from build123d import *

# Parameters (mm, degrees)
F0_W          = 76.2
F0_H          = 12.7
F1_DEPTH      = 19.05
F2_R          = 19.05
F3_DEPTH      = 19.05
F3_DEPTH_BACK = 8.2509537059
F4_START      = 20.9509537059
F4_DEPTH      = 23.4990462941
F5_R          = 7.9375
F6_DEPTH      = 101.6
F8_START      = 23.32678
F7_R          = 12.7
F8_DEPTH      = 6.84063


with BuildPart() as f1:
    # F0 (on Front) → F1 (new body, symmetric)
    with BuildSketch(Plane.XZ):
        with Locations((1.1919587851, 14.6009537059)):
            Rectangle(F0_W, F0_H)
    extrude(amount=F1_DEPTH, both=True)

    # F2 (on Top) → F3 (join, two sides)
    with BuildSketch(Plane.XY) as f3_sk:
        Circle(F2_R)
    extrude(amount=-F3_DEPTH)
    extrude(f3_sk.sketch, amount=F3_DEPTH_BACK)

    # F2 (on Top) → F4 (join)
    with BuildSketch(Plane.XY.offset(F4_START)):
        Circle(F2_R)
    extrude(amount=F4_DEPTH)

    # F5 (on Top) → F6 (cut, symmetric)
    with BuildSketch(Plane.XY):
        Circle(F5_R)
    extrude(amount=F6_DEPTH, both=True, mode=Mode.SUBTRACT)

    # F7 (on Top) → F8 (cut)
    with BuildSketch(Plane.XY.offset(F8_START)):
        Circle(F7_R)
    extrude(amount=F8_DEPTH, mode=Mode.SUBTRACT)


solid = f1.part
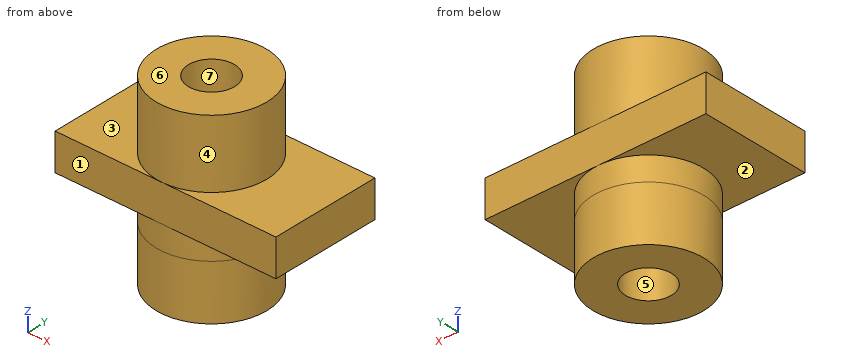
Can you work these out from the model? Positions are in its coordinate system, mm. Face numbers are marked on the shaded views. A direction names the side the tool comes from. Give positions to 0.01 mm unless a question says otherwise; leave off trailing zeros. Order: outer loops, then holes, each group sorted by start corner. A loop starts at its lowest first (then second) coordinate and runs counter-clockwise, first axis right, second up. Notation, with made-up numbers: M -33.75,8 L -7.75,8 A27 ccw -7.75,37 Z; hole C 55,67 d9. An arc over 180 degrees is marked long. Use one line per item in the form item = value. Start each with the question number.
Item 1: Will these pins go through, and if not, where does the flat tip stop? pin 1 Ø1 at (y, z) = (6.5, -1.5) entering from +X; pin 2 Ø20.5 at (x, y) = (0, 0) entering from -Z; pin 3 Ø1.5 at (y, z) = (4, 2) entering from -X; pin 4 Ø4 at (x, z) = (-16, 35) entering from +Y.
Item 2: If we section it at C-C (z = 25): Write out the boundary of the cut face in (x, y).
Item 3: If we section it at A-A (y = 3.5): Write out the boundary of the cut face in (x, z), then the cut area to 3 significant figures.
Item 4: If we section it at B-B (x = 2): Write out the boundary of the cut face in (y, z).
Item 5: We'd pull the mould along X, two halves only. Please class the marked faces 4, 5, 6 and 7: +X half, -X half, draft (parallel to the pull), parting line (faces both ways), or undercut.
Item 6: If I drill on line 1 along Y through (x, z) = (0, 11.5); line 2 along Y through (x, z) = (0, 28.5); line 3 along Z through (x, y) = (-23, -4), over which ranges is the centre line in solid material (lowest first)?
Item 7: If we section it at D-D (x = -30): Write out the boundary of the cut face in (y, z).
Item 8: For the marked faces 1, 2 and 3, which set-ups out of +Z, -Z, +X, -X, +Y, -Y let a thin tool reach every point of the face, with its end or its side?
Outcome:
q1.pin_1 = 18.08
q1.pin_2 = -19.05
q1.pin_3 = -18.77
q1.pin_4 = 12.92
q2.outline = C 0,0 d38.1; hole C 0,0 d25.4
q3.outline = M -36.91,8.25 L -18.73,8.25 L -18.73,-19.05 L -7.12,-19.05 L -7.12,23.33 L -12.21,23.33 L -12.21,30.17 L -7.12,30.17 L -7.12,44.45 L -18.73,44.45 L -18.73,20.95 L -36.91,20.95 Z; M 7.12,-19.05 L 18.73,-19.05 L 18.73,8.25 L 39.29,8.25 L 39.29,20.95 L 18.73,20.95 L 18.73,44.45 L 7.12,44.45 L 7.12,30.17 L 12.21,30.17 L 12.21,23.33 L 7.12,23.33 Z
q3.area = 1,900 mm2
q4.outline = M -19.05,8.25 L -18.94,8.25 L -18.94,-19.05 L -7.68,-19.05 L -7.68,23.33 L -12.54,23.33 L -12.54,30.17 L -7.68,30.17 L -7.68,44.45 L -18.94,44.45 L -18.94,20.95 L -19.05,20.95 Z; M 7.68,-19.05 L 18.94,-19.05 L 18.94,8.25 L 19.05,8.25 L 19.05,20.95 L 18.94,20.95 L 18.94,44.45 L 7.68,44.45 L 7.68,30.17 L 12.54,30.17 L 12.54,23.33 L 7.68,23.33 Z
q5.face_4 = parting line
q5.face_5 = undercut
q5.face_6 = draft
q5.face_7 = undercut
q6.line_1 = -19.05 to -7.94, 7.94 to 19.05
q6.line_2 = -19.05 to -12.7, 12.7 to 19.05
q6.line_3 = 8.25 to 20.95
q7.outline = M -19.05,8.25 L 19.05,8.25 L 19.05,20.95 L -19.05,20.95 Z
q8.face_1 = +Z, -Z, +X, -X, -Y
q8.face_2 = -Z, -X
q8.face_3 = +Z, -X
